from build123d import *

# Parameters (mm, degrees)
F1_DEPTH = 15
F2_R     = 2.1
F3_DEPTH = 5
F4_R     = 2.295
F5_DEPTH = 38.251
F6_R     = 2.6
F6_R_2   = 2.295
F7_DEPTH = 3
F8_SIZE  = 2
F9_SIZE  = 1


with BuildPart() as f1:
    # F0 (on Front) → F1 (new body)
    with BuildSketch(Plane.XZ):
        with BuildLine():
            ThreePointArc((0, 5), (1.464466, 1.464466), (5, 0))
            Line((5, 0), (38.25, 0))
            Line((38.25, 0), (38.25, 5))
            Line((38.25, 5), (17, 5))
            Line((17, 5), (17, 17))
            Line((17, 17), (27, 17))
            Line((27, 17), (27, 32))
            Line((27, 32), (14.5, 32))
            Line((14.5, 32), (14.5, 19))
            Line((14.5, 19), (3, 19))
            Line((3, 19), (3, 32))
            Line((3, 32), (0, 32))
            Line((0, 32), (0, 5))
        make_face()
    extrude(amount=F1_DEPTH)

    # F2 (on face) → F3 (cut, through all)
    with BuildSketch(Plane(origin=(0, 0, 0), x_dir=(1, 0, 0), z_dir=(0, 0, -1))):
        with Locations((29, 7.5)):
            Circle(F2_R)
    extrude(amount=-F3_DEPTH, mode=Mode.SUBTRACT)

    # F4 (on face) → F5 (cut, through all)
    with BuildSketch(Plane(origin=(0, 0, 0), x_dir=(0, -1, 0), z_dir=(-1, 0, 0))):
        with Locations((7.5, 25.5)):
            Circle(F4_R)
    extrude(amount=-F5_DEPTH, mode=Mode.SUBTRACT)

    # F6 (on face) → F7 (cut, through all)
    with BuildSketch(Plane(origin=(0, 0, 0), x_dir=(0, -1, 0), z_dir=(-1, 0, 0))):
        with Locations((7.5, 25.5)):
            Circle(F6_R)
        with Locations((7.5, 25.5)):
            Circle(F6_R_2, mode=Mode.SUBTRACT)
    extrude(amount=-F7_DEPTH, mode=Mode.SUBTRACT)

    # F8
    f8_edges = [f1.edges().sort_by_distance(p)[0] for p in [
        (27, -7.5, 32),
        (0, -7.5, 32),
    ]]
    chamfer(f8_edges, length=F8_SIZE)

    # F9
    f9_edges = [f1.edges().sort_by_distance(p)[0] for p in [
        (3, -7.5, 19),
        (14.5, -7.5, 19),
    ]]
    chamfer(f9_edges, length=F9_SIZE)


solid = f1.part
Can you work these out from the model? Positions are in its coordinate system, mm. A direction names the side the tool comes from. Coordinates: 2 decimals unless noted, no trailing zeros. Write each loop counter-clockwise with the first axis right and the second up, starting at its lowest first coordinate (ties: lowest second). Pieces come first, ordered by that corner, then holes. Notation, with made-up numbers: (35, 15) -> (75, 15) arc R16 cw to (75, 19) -> close; hole circle Ø10 at (1, 70.5). An arc over 180 degrees is marked (long way). Write each question's results on one line, items separated by ' | '. Start each with the question number.
Item 1: Please list where these lines run through material, in increasing order: probe 1 along Z at (x, y) = (19.75, -7.5) (3 decimals); probe 2 along X at (y, z) = (-2.5, 29); probe 3 along Z at (x, y) = (19, -10.5).
Item 2: On a 3-axis mill with a long thin cutter (end or side, diameter ignored), from which of +Z, -Z, +X, -X, +Y, -Y can I reach the whole of each face in a straight line? I mean faces 5 (the flat face through (38.25, -7, 2)), 6 (the flat face through (14, -7.4, 19.5)), 7 (the flat face through (22, -7, 17)), 8 (the flat face through (0, -7, 18)), 9 (the flat face through (27, -7, 22)). Say none if no direction works.
Item 3: If we section it at B-B, the plane z = 25.5: Write out the boundary of the cut face in (x, y) (3 decimals), and give its area (3 significant figures).
Item 4: If we section it at A-A, the plane x = 17.5: Write out the boundary of the cut face in (y, z) (3 decimals).
Item 5: I'm going to push flat-ended pins straight in: P1, Ø4.5, axis at x = 27.5, y = -5.5, coming from the +Z side; P2, Ø6.5, axis at y = -10.5, z = 21, coming from the +X side; P3, Ø3.5, axis at y = -9, z = 12.5, coming from the +X side. Where does each tip first touch, or does it pass through?
Item 6: If we section it at D-D, the plane x = 29: Write out the boundary of the cut face in (y, z).
Item 7: If we section it at C-C, the plane y = -7.5: Count the separate pieces of the cut face and the enclosed holes in it, and give its area (3 significant figures).
Item 8: Thinking about a two-plate mould opening in Y: for faces 1 (the cylindrical face through (1.479, -7.162, 28.078)), 2 (the flat face through (9, -7, 19)), 3 (the cylindrical face through (27.452, -8.919, 2.465)), 4 (the flat face through (15, 0, 16)), which applies, released by +Y, released by -Y, zero draft, split by the parting line, or undercut?
Answer block:
1) probe 1: 0 to 5, 17 to 23.205, 27.795 to 32 | probe 2: 0 to 3, 14.5 to 27 | probe 3: 0 to 5, 17 to 32
2) face 5: +Z, -Z, +X, +Y, -Y | face 6: +Z, +Y, -Y | face 7: +X, +Y, -Y | face 8: +Z, -Z, -X, +Y, -Y | face 9: +Z, +X, +Y, -Y
3) outline: (0, -15) -> (3, -15) -> (3, -10.1) -> (0, -10.1) -> close; (0, -4.9) -> (3, -4.9) -> (3, 0) -> (0, 0) -> close; (14.5, -15) -> (27, -15) -> (27, -9.795) -> (14.5, -9.795) -> close; (14.5, -5.205) -> (27, -5.205) -> (27, 0) -> (14.5, 0) -> close | area: 160 mm²
4) outline: (-15, 0) -> (0, 0) -> (0, 5) -> (-15, 5) -> close; (-15, 17) -> (0, 17) -> (0, 32) -> (-15, 32) -> close; hole circle Ø4.59 at (-7.5, 25.5)
5) P1: z = 31.75 | P2: x = 27 | P3: x = 17
6) outline: (-15, 0) -> (-9.6, 0) -> (-9.6, 5) -> (-15, 5) -> close; (-5.4, 0) -> (0, 0) -> (0, 5) -> (-5.4, 5) -> close
7) separate pieces: 4 | enclosed holes: 0 | area: 548 mm²
8) face 1: undercut | face 2: zero draft | face 3: undercut | face 4: released by +Y
